```python
from build123d import *

# Parameters (mm, degrees)
SKETCH1_W           = 110
SKETCH1_H           = 2.5
SKETCH1_W_2         = 10
BOSS_EXTRUDE1_DEPTH = 2.5


with BuildPart() as part:
    # Sketch1 → Boss-Extrude1 (new body)
    with BuildSketch(Plane.XY):
        Polygon((-65, -12.5), (65, -12.5), (65, -5), (57.5, -5), (57.5, -2.5), (65, -2.5), (65, 0), (57.5, 0), (57.5, 2.5), (65, 2.5), (65, 5), (57.5, 5), (57.5, 7.5), (65, 7.5), (65, 10), (57.5, 10), (57.5, 12.5), (55, 12.5), (55, 10), (-55, 10), (-55, 12.5), (-57.5, 12.5), (-57.5, 10), (-65, 10), (-65, 7.5), (-57.5, 7.5), (-57.5, 5), (-65, 5), (-65, 2.5), (-57.5, 2.5), (-57.5, 0), (-65, 0), (-65, -2.5), (-57.5, -2.5), (-57.5, -5), (-65, -5), align=None)
        with Locations((0, -3.75)):
            Rectangle(SKETCH1_W, SKETCH1_H, mode=Mode.SUBTRACT)
        with Locations((0, 6.25)):
            Rectangle(SKETCH1_W, SKETCH1_H, mode=Mode.SUBTRACT)
        with Locations((0, 1.25)):
            Rectangle(SKETCH1_W, SKETCH1_H, mode=Mode.SUBTRACT)
        with Locations((-15, -8.75)):
            Rectangle(SKETCH1_W_2, SKETCH1_H, mode=Mode.SUBTRACT)
        with Locations((-35, -8.75)):
            Rectangle(SKETCH1_W_2, SKETCH1_H, mode=Mode.SUBTRACT)
        with Locations((15, -8.75)):
            Rectangle(SKETCH1_W_2, SKETCH1_H, mode=Mode.SUBTRACT)
        with Locations((35, -8.75)):
            Rectangle(SKETCH1_W_2, SKETCH1_H, mode=Mode.SUBTRACT)
    extrude(amount=BOSS_EXTRUDE1_DEPTH)


solid = part.part
```
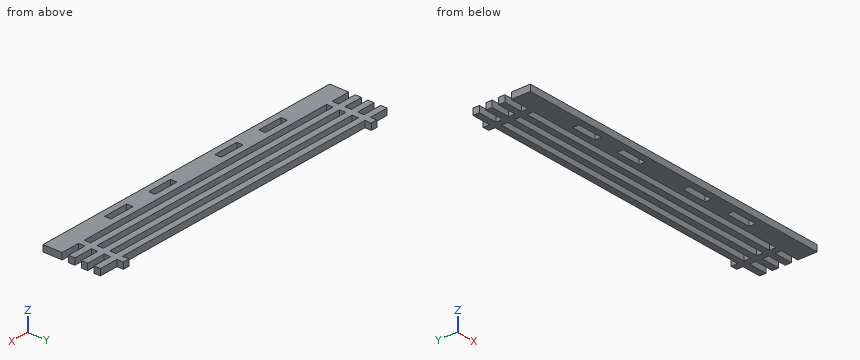
Build history of the part. All positions in model axes, mm. Give positions to 0.01 mm unless a question says otherwise; leave off trailing zeros. Loops run counter-clockwise (first coordinate to the right, second up) from the corner with the lowest first, then second, coordinate; pieces in that order, holes last.
Item 1: Drill centre lines: line 1 (Y direction, x = 53, z = 0.8); line 2 (Y direction, x = 39, z = 2.25); line 3 (X direction, y = -3.5, z = 0.1). Where is each one in solid material? Low to high.
Answers follow:
line 1: y = -12.5 to -5, -2.5 to 0, 2.5 to 5, 7.5 to 10
line 2: y = -12.5 to -10, -7.5 to -5, -2.5 to 0, 2.5 to 5, 7.5 to 10
line 3: x = -57.5 to -55, 55 to 57.5
Item 2: Slice it at B-B, the plane x = 12. List the corners of the cut face in (y, z).
Answers follow:
outline: (-12.5, 0) - (-10, 0) - (-10, 2.5) - (-12.5, 2.5) - close; (-7.5, 0) - (-5, 0) - (-5, 2.5) - (-7.5, 2.5) - close; (-2.5, 0) - (0, 0) - (0, 2.5) - (-2.5, 2.5) - close; (2.5, 0) - (5, 0) - (5, 2.5) - (2.5, 2.5) - close; (7.5, 0) - (10, 0) - (10, 2.5) - (7.5, 2.5) - close
Item 3: Slice it at C-C, the plane z = 2. Give the number of separate pieces and of enclosed holes in the cut face, and give its area (3 significant figures).
Answers follow:
separate pieces: 1
enclosed holes: 7
area: 1,900 mm2
Item 4: Flat gauge pins, fed straight in: pin 1 (0.8 mm diameter, centred on x = -35.5, z = 1, fed in from +Y); pin 2 (1.2 mm diameter, centred on y = 6, z = 1.5, fed in from -X); pin 3 (2 mm diameter, centred on x = -2.5, y = -7.5, fed in from -Z). Where does each tip first touch, or does it go through?
Answers follow:
pin 1: stops at y = 10
pin 2: stops at x = -57.5
pin 3: stops at z = 0
Item 5: Slice it at A-A, the plane x = 49. List the corners of the cut face in (y, z).
Answers follow:
outline: (-12.5, 0) - (-5, 0) - (-5, 2.5) - (-12.5, 2.5) - close; (-2.5, 0) - (0, 0) - (0, 2.5) - (-2.5, 2.5) - close; (2.5, 0) - (5, 0) - (5, 2.5) - (2.5, 2.5) - close; (7.5, 0) - (10, 0) - (10, 2.5) - (7.5, 2.5) - close
